```python
from build123d import *

# Parameters (mm, degrees)
BOSS_EXTRUDE1_DEPTH = 101.6


with BuildPart() as part:
    # Sketch1 → Boss-Extrude1 (new body)
    with BuildSketch(Plane.XY):
        with BuildLine():
            Line((-111.087162468, 18.269301554), (-111.087162468, -32.530698446))
            Line((-111.087162468, -32.530698446), (-85.687162468, -32.530698446))
            ThreePointArc((-85.687162468, -32.530698446), (-78.24767471, -14.570186204), (-60.287162468, -7.130698446))
            ThreePointArc((-60.287162468, -7.130698446), (-42.326650226, -14.570186204), (-34.887162468, -32.530698446))
            Line((-34.887162468, -32.530698446), (15.912837532, -32.530698446))
            Line((15.912837532, -32.530698446), (66.712837532, -32.530698446))
            Line((66.712837532, -32.530698446), (92.112837532, -32.530698446))
            Line((92.112837532, -32.530698446), (92.112837532, 18.269301554))
            Line((92.112837532, 18.269301554), (66.712837532, 18.269301554))
            Line((66.712837532, 18.269301554), (41.312837532, 69.069301554))
            Line((41.312837532, 69.069301554), (-60.287162468, 69.069301554))
            Line((-60.287162468, 69.069301554), (-85.687162468, 18.269301554))
            Line((-85.687162468, 18.269301554), (-111.087162468, 18.269301554))
        make_face()
    extrude(amount=BOSS_EXTRUDE1_DEPTH)


solid = part.part
```
Here's how the part is built. I have some questions about the finished solid (model axes, mm). A direction names the side the tool comes from. Coordinates: 2 decimals unless noted, no trailing zeros. Order: outer loops, then holes, each group sorted by start corner. A loop starts at its lowest first (then second) coordinate and runs counter-clockwise, first axis right, second up.
Item 1: If we section it at B-B, the plane z = 68: List the corners of the cut face in (x, y) for me, then the cut area to 3 significant figures.
Response values:
outline: (-111.09, -32.53) - (-85.69, -32.53) arc R25.4 cw to (-34.89, -32.53) - (92.11, -32.53) - (92.11, 18.27) - (66.71, 18.27) - (41.31, 69.07) - (-60.29, 69.07) - (-85.69, 18.27) - (-111.09, 18.27) - close
area: 15,800 mm2
Item 2: I need wall thicknesses on probe 1 along Y at (x, z) = (-95.5, 55.5); probe 2 along X at (y, z) = (-21.5, 57); probe 3 along X at (y, z) = (-20, 45). Which ranges of each line are inside material? Lowest first, please.
Response values:
probe 1: y = -32.53 to 18.27
probe 2: x = -111.09 to -83.17, -37.41 to 92.11
probe 3: x = -111.09 to -82.38, -38.19 to 92.11
Item 3: If we section it at A-A, the plane y = -17: List the corners of the cut face in (x, z) for me.
Response values:
outline: (-111.09, 0) - (-80.39, 0) - (-80.39, 101.6) - (-111.09, 101.6) - close; (-40.19, 0) - (92.11, 0) - (92.11, 101.6) - (-40.19, 101.6) - close
Item 4: If we section it at D-D, the plane y = 32.5: List the corners of the cut face in (x, z) for me.
Response values:
outline: (-78.57, 0) - (59.6, 0) - (59.6, 101.6) - (-78.57, 101.6) - close
Item 5: I'm going to push flat-ended pins straight in: pin 1 Ø20.5 at (x, z) = (-93.5, 54.5) entering from +Y; pin 2 Ø7.5 at (x, z) = (81.5, 28.5) entering from +Y; pin 3 Ø6 at (y, z) = (39, 84) entering from +X. Where does each tip first touch, or does it pass through?
Response values:
pin 1: stops at y = 23.14
pin 2: stops at y = 18.27
pin 3: stops at x = 57.85
Item 6: Which directions (+Z, -Z, +X, -X, +Y, -Y) give clear straight access to the entire face, cutting with the end or side of a thin tool? Please do faces 1 (the face through (-99, -32.531, 50)), 2 (the face through (-98, 18.269, 50)), 3 (the face through (80, 18.269, 50)).
Response values:
face 1: +Z, -Z, +X, -X, -Y
face 2: +Z, -Z, -X, +Y
face 3: +Z, -Z, +X, +Y
Item 7: If we section it at C-C, the plane x = 73: List the corners of the cut face in (y, z) for me.
Response values:
outline: (-32.53, 0) - (18.27, 0) - (18.27, 101.6) - (-32.53, 101.6) - close
